Could you check a few things on this model? Use its own coordinates, in mm. A direction names the side the tool comes from. Coordinates: 2 decimals unless noted, no trailing zeros. Write each loop counter-clockwise with the first axis right and the second up, starting at its lowest first coordinate (ties: lowest second). Pieces come first, ordered by that corner, then holes. Notation, with made-up numbers: (14, -13.5) - (46, -13.5) arc R37 ccw to (46, 22.5) - close; hole circle Ø2 at (82.25, 36.25). An arc over 180 degrees is marked (long way). Answer as a JSON object with one key per item and string values. Group by question number.
1) On a 3-axis mill with a long thin cutter (end or side, diameter ignored), from which of +Z, -Z, +X, -X, +Y, -Y can I reach the whole of each face in a straight line? I mean faces 4 (the flat face through (-6, 2.6, -1)), 5 (the flat face through (-7, 5.01, 0.18)), 6 (the flat face through (-4.4, 5, -1)), 7 (the flat face through (-6, 7.5, 0)). Say none if no direction works.
2) If we section it at C-C (y = 8): Write out the boundary of the cut face in (x, z).
3) Please list where these lines run through material, in increasing order: line 1 along Z through (x, y) = (-3, 14.25); line 2 along X through (y, z) = (7, -0.6); line 3 along Y through (x, z) = (-5.5, -1.4).
4) If we section it at A-A (z = 1.95): Write out the boundary of the cut face in (x, y).
5) Will these pins go through, and if not, where does the flat tip stop? pin 1 Ø2 at (x, y) = (-8.5, 7) entering from -Z; pin 2 Ø1.1 at (y, z) = (6, -1) entering from +X; pin 3 Ø3 at (x, z) = (-5, -0.5) entering from +Y.
6) If we section it at B-B (x = -6): Write out the boundary of the cut face in (y, z).
7) We'd pull the mould along Z, two halves only. Please class faces 1 (the flat face through (-6, 15, 2)), 2 (the cylindrical face through (-5.784, 2.299, 0.966)), 3 (the flat face through (-4.6, 5.01, 0.19)): released by +Z, released by -Z, zero draft, split by the parting line, or undercut.
8) If we section it at D-D (z = -1): Write out the boundary of the cut face in (x, y), plus the area to 3 significant figures.
```python
from build123d import *

# Parameters (mm, degrees)
SKETCH2_W           = 10
SKETCH2_H           = 2
BOSS_EXTRUDE1_DEPTH = 15
BOSS_EXTRUDE2_DEPTH = 4.9
FILLET1_R           = 2
FILLET2_R           = 1


with BuildPart() as part:
    # Sketch2 → Boss-Extrude1 (new body)
    with BuildSketch(Plane(origin=(0, 0, 0), x_dir=(1, 0, 0), z_dir=(0, 1, 0))):
        with Locations((-5.80018665, -2.25133902)):
            Rectangle(SKETCH2_W, SKETCH2_H)
    extrude(amount=BOSS_EXTRUDE1_DEPTH)

    # Sketch3 → Boss-Extrude2 (add)
    with BuildSketch(Plane(origin=(0, 7.5, 0), x_dir=(-1, 0, 0), z_dir=(0, -1, 0))):
        Polygon((4.80018665, -1.437939643), (4.80018665, -0.785111254), (4.40018665, 0.414888746), (4.40018665, 1.79866098), (7.20018665, 1.79866098), (7.20018665, 0.414888746), (6.80018665, -0.785111254), (6.80018665, -1.437939643), align=None)
    extrude(amount=BOSS_EXTRUDE2_DEPTH)

    # Fillet1
    fillet1_edges = [part.edges().sort_by_distance(p)[0] for p in [
        (-10.80018665, 15, 2.25133902),
        (-0.80018665, 15, 2.25133902),
        (-10.80018665, 0, 2.25133902),
        (-0.80018665, 0, 2.25133902),
    ]]
    fillet(fillet1_edges, radius=FILLET1_R)

    # Fillet2
    fillet2_edges = [part.edges().sort_by_distance(p)[0] for p in [
        (-5.80018665, 2.6, 1.25133902),
    ]]
    fillet(fillet2_edges, radius=FILLET2_R)


solid = part.part
```
Here are the results:
{
 "1": {"face 4": "-Z, +X, -X, -Y", "face 5": "-X, +Y, -Y", "face 6": "-Z, +X, +Y, -Y", "face 7": "-Z, +X, -X, +Y"},
 "2": {"outline": "(-10.8, 1.25) - (-0.8, 1.25) - (-0.8, 3.25) - (-10.8, 3.25) - close"},
 "3": {"line 1": "z = 1.25 to 3.25", "line 2": "x = -7.2 to -4.4", "line 3": "y = 2.6 to 7.5"},
 "4": {"outline": "(-10.8, 2) arc R2 ccw to (-8.8, 0) - (-2.8, 0) arc R2 ccw to (-0.8, 2) - (-0.8, 13) arc R2 ccw to (-2.8, 15) - (-8.8, 15) arc R2 ccw to (-10.8, 13) - close"},
 "5": {"pin 1": "stops at z = 1.25", "pin 2": "stops at x = -4.4", "pin 3": "stops at y = 7.5"},
 "6": {"outline": "(0, 1.25) - (1.6, 1.25) arc R1 cw to (2.6, 0.25) - (2.6, -1.8) - (7.5, -1.8) - (7.5, 1.25) - (15, 1.25) - (15, 3.25) - (0, 3.25) - close"},
 "7": {"face 1": "zero draft", "face 2": "released by -Z", "face 3": "undercut"},
 "8": {"outline": "(-7.2, 2.6) - (-4.4, 2.6) - (-4.4, 7.5) - (-7.2, 7.5) - close", "area": "13.7 mm²"}
}
